from build123d import *

# Parameters (mm, degrees)
PAD_DEPTH    = 30
SKETCH001_R  = 5
POCKET_DEPTH = 50.001


with BuildPart() as part:
    # Sketch → Pad (new body)
    with BuildSketch(Plane.XZ):
        with BuildLine():
            Line((0, 0), (100, 0))
            Line((100, 0), (100, 30))
            ThreePointArc((100, 30), (94.142136, 44.142136), (80, 50))
            Line((60, 50), (80, 50))
            Line((0, 15.358984), (60, 50))
            Line((0, 0), (0, 15.358984))
        make_face()
    extrude(amount=-PAD_DEPTH)

    # Sketch001 (on DatumPlane) → Pocket (cut, through all)
    with BuildSketch(Plane(origin=(70, 15, 50), x_dir=(1, 0, 0), z_dir=(0, 0, 1))):
        Circle(SKETCH001_R)
    extrude(amount=-POCKET_DEPTH, mode=Mode.SUBTRACT)


solid = part.part
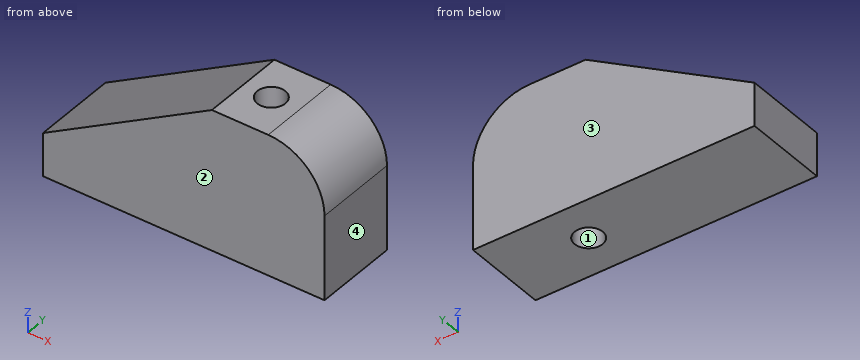
Geometry check sheet. Reference: the model listing, model coordinates, mm. Face numbers are marked on the shaded views. Coordinates: 2 decimals unless noted, no trailing zeros. Order: outer loops, then holes, each group sorted by start corner. A loop starts at its lowest first (then second) coordinate and runs counter-clockwise, first axis right, second up. Notation, with made-up numbers: (40, 1.5) - (53, 1.5) arc R16 ccw to (53, 9.5) - close; hole circle Ø9 at (87.5, 12). An arc over 180 degrees is marked (long way). Answer in a Markdown table with one row per item. Add a question column.
1) Cross-section at C-C, the plane z = 12. Record the cut outline in (x, y), then the cut area to 3 significant figures.
2) Cross-section at D-D, the plane y = 3. Record the cut outline in (x, z).
3) Material ranges on line 1 along Y through (x, z) = (70, 32); line 2 along X through (y, z) = (14.75, 15); line 3 along Y through (x, z) = (68.5, 4), recorded low to high. Write a range as [from, to].
4) Gauge pin test, flat ends, axial feed: P1, Ø9, axis at x = 70, y = 15, coming from the -Z side; P2, Ø8, axis at x = 26, y = 21.5, coming from the +Z side; P3, Ø6, axis at x = 17.5, y = 23, coming from the +Z side. Record the tip position at first contact, or that the pin passes through.
5) Cross-section at B-B, the plane y = 11. Record the cut outline in (x, z), then the cut area to 3 significant figures.
6) Release check for a two-part mould opening along Y. For the marked faces 1, 2, 3 and 4 record: +Y half, -Y half, draft (parallel to the pull), parting line (faces both ways), or undercut.
7) Cross-section at A-A, the plane x = 70. Record the cut outline in (y, z).
Check result:
| question | item | result |
|---|---|---|
| 1 | outline | (0, 0) - (100, 0) - (100, 30) - (0, 30) - close; hole circle Ø10 at (70, 15) |
| 1 | area | 2,920 mm² |
| 2 | outline | (0, 0) - (100, 0) - (100, 30) arc R20 ccw to (80, 50) - (60, 50) - (0, 15.36) - close |
| 3 | line 1 | y = [0, 10], [20, 30] |
| 3 | line 2 | x = [0, 65.01], [74.99, 100] |
| 3 | line 3 | y = [0, 10.23], [19.77, 30] |
| 4 | P1 | passes through |
| 4 | P2 | stops at z = 32.68 |
| 4 | P3 | stops at z = 27.19 |
| 5 | outline | (0, 0) - (67, 0) - (67, 50) - (60, 50) - (0, 15.36) - close; (73, 0) - (100, 0) - (100, 30) arc R20 ccw to (80, 50) - (73, 50) - close |
| 5 | area | 3,570 mm² |
| 6 | face 1 | undercut |
| 6 | face 2 | -Y half |
| 6 | face 3 | +Y half |
| 6 | face 4 | draft |
| 7 | outline | (0, 0) - (10, 0) - (10, 50) - (0, 50) - close; (20, 0) - (30, 0) - (30, 50) - (20, 50) - close |
